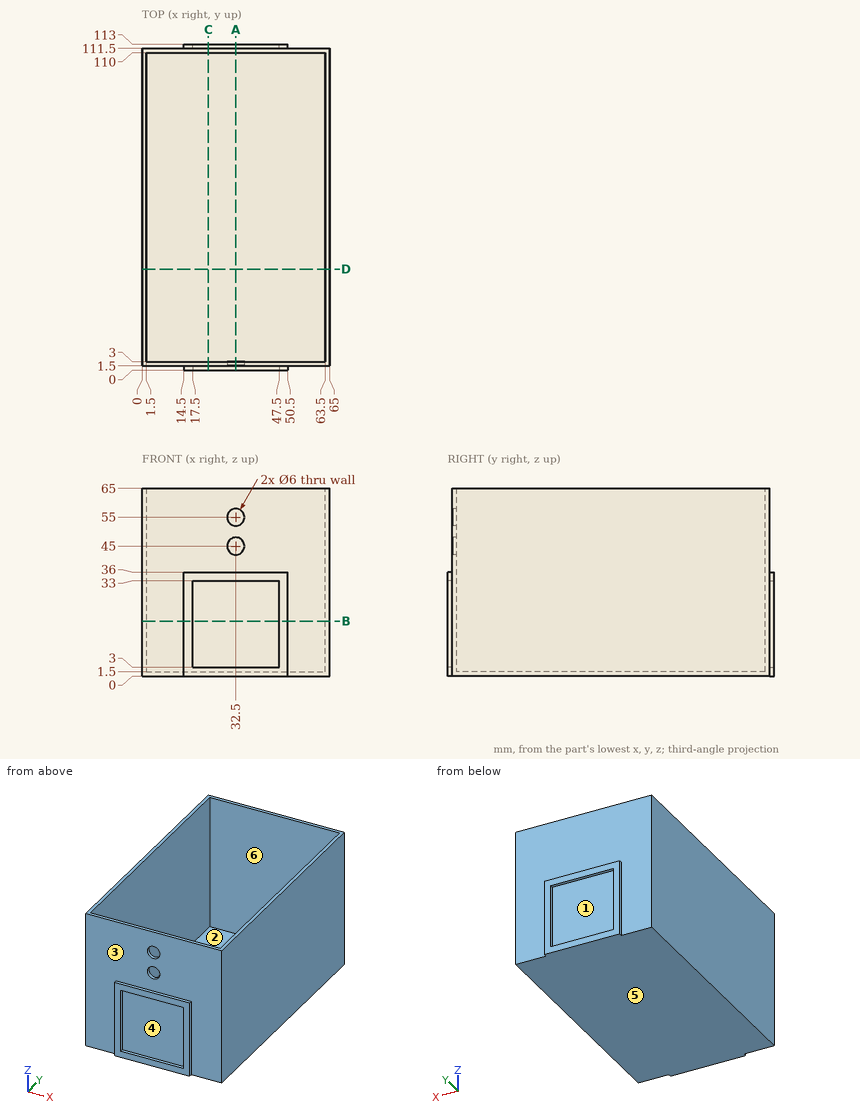
Source: three-view drawing plus pictorial views. Frame: mm from the lowest corner of the part. A direction names the side the tool comes from. Coordinates: 2 decimals unless noted, no trailing zeros. Loops run counter-clockwise (first coordinate to the right, second up) from the corner with the lowest first, then second, coordinate; pieces in that order, holes last. Notation, with made-up numbers: (35.5, 6.5) - (48.5, 6.5) arc R26 cw to (48.5, 35.5) - close; hole circle Ø9 at (-5.75, -12). An arc over 180 degrees is marked (long way). Answer in a Markdown table with one row per item. Add a question column.
Item 1: Access query for the marked faces 4, 5 and 6. Directions: +Z, -Z, +X, -X, +Y, -Y. A direction counts if a zero-diameter tool reaches every point of the face in a straight line with its end or side. Return the directions, or none.
Item 2: Section query B-B on z = 19. Return the cut outline in (x, y), then the cut area to 3 significant figures.
Item 3: Section query D-D on y = 35. Return the cut outline in (x, z), then the cut area to 3 significant figures.
Item 4: Section query C-C on x = 23. Return the cut outline in (y, z).
Item 5: Section query A-A on x = 32.5. Return the cut outline in (y, z).
Item 6: Line query: line 1 along Z through (x, y) = (32.5, 1.85); line 2 along Y through (x, z) = (24, 15); line 3 along Z through (x, y) = (55, 68.5). Output: solid intervals per line, ascending. Write a range as [from, to].
Item 7: Mould query, pull axis Z, two halves, no side actions, for the marked faces 1, 2 and 3. Classes: released by +Z, released by -Z, zero draft, split by the parting line, or undercut.
Item 8: Contact query for flat-ended pins moving along their axis: P1, Ø1.2, axis at x = 26.5, y = 0.5, coming from the +Z side; P2, Ø5, axis at x = 36, z = 16, coming from the +Y side; P3, Ø5, axis at x = 12.5, y = 98, coming from the +Z side. Output: stop coordinate, or through.
Recorded:
| question | item | result |
|---|---|---|
| 1 | face 4 | -Y |
| 1 | face 5 | -Z, +X, -X, +Y, -Y |
| 1 | face 6 | +Z |
| 2 | outline | (0, 1.5) - (14.5, 1.5) - (14.5, 0) - (17.5, 0) - (17.5, 1.5) - (47.5, 1.5) - (47.5, 0) - (50.5, 0) - (50.5, 1.5) - (65, 1.5) - (65, 111.5) - (50.5, 111.5) - (50.5, 113) - (47.5, 113) - (47.5, 111.5) - (17.5, 111.5) - (17.5, 113) - (14.5, 113) - (14.5, 111.5) - (0, 111.5) - close; hole (1.5, 3) - (63.5, 3) - (63.5, 110) - (1.5, 110) - close |
| 2 | area | 534 mm^2 |
| 3 | outline | (0, 0) - (65, 0) - (65, 65) - (63.5, 65) - (63.5, 1.5) - (1.5, 1.5) - (1.5, 65) - (0, 65) - close |
| 3 | area | 288 mm^2 |
| 4 | outline | (0, 0) - (113, 0) - (113, 3) - (111.5, 3) - (111.5, 33) - (113, 33) - (113, 36) - (111.5, 36) - (111.5, 65) - (110, 65) - (110, 1.5) - (3, 1.5) - (3, 65) - (1.5, 65) - (1.5, 36) - (0, 36) - (0, 33) - (1.5, 33) - (1.5, 3) - (0, 3) - close |
| 5 | outline | (0, 0) - (113, 0) - (113, 3) - (111.5, 3) - (111.5, 33) - (113, 33) - (113, 36) - (111.5, 36) - (111.5, 65) - (110, 65) - (110, 1.5) - (3, 1.5) - (3, 42) - (1.5, 42) - (1.5, 36) - (0, 36) - (0, 33) - (1.5, 33) - (1.5, 3) - (0, 3) - close; (1.5, 48) - (3, 48) - (3, 52) - (1.5, 52) - close; (1.5, 58) - (3, 58) - (3, 65) - (1.5, 65) - close |
| 6 | line 1 | [0, 42], [48, 52], [58, 65] |
| 6 | line 2 | [1.5, 3], [110, 111.5] |
| 6 | line 3 | [0, 1.5] |
| 7 | face 1 | undercut |
| 7 | face 2 | released by +Z |
| 7 | face 3 | zero draft |
| 8 | P1 | z = 36 |
| 8 | P2 | y = 111.5 |
| 8 | P3 | z = 1.5 |
